For this review, take the finished solid that the model builds, in its own axes (mm). Face numbers are marked on the shaded views. A direction names the side the tool comes from. Give positions to 0.01 mm unless a question says otherwise; leave off trailing zeros. Write each loop counter-clockwise with the first axis right and the second up, starting at its lowest first coordinate (ties: lowest second). Pieces come first, ordered by that corner, then holes. Notation, with made-up numbers: (89.25, 63.5) -> (134.25, 63.5) arc R28 ccw to (134.25, 84.5) -> close; hole circle Ø8 at (72.5, 43). An arc over 180 degrees is marked (long way). Return JSON: item names as keys, results as strings.
from build123d import *

# Parameters (mm, degrees)
SKETCH1_W           = 12
SKETCH1_H           = 16
SKETCH1_R           = 2.1
SKETCH1_W_2         = 2
BOSS_EXTRUDE1_DEPTH = 20
FILLET1_R           = 5
SKETCH2_W           = 9
SKETCH2_H           = 1.9
BOSS_EXTRUDE2_DEPTH = 5


with BuildPart() as part:
    # Sketch1 → Boss-Extrude1 (new body)
    # profile 1 of 2: a face of its own
    with BuildSketch(Plane(origin=(0, 0, 0), x_dir=(1, 0, 0), z_dir=(0, 1, 0))):
        Rectangle(SKETCH1_W, SKETCH1_H)
        with Locations(Location((0, 0, 0), (0, 0, 270))):
            Circle(SKETCH1_R, mode=Mode.SUBTRACT)
    # profile 2 of 2: a face of its own
    with BuildSketch(Plane(origin=(0, 0, 0), x_dir=(1, 0, 0), z_dir=(0, 1, 0))):
        with Locations((7, 0)):
            Rectangle(SKETCH1_W_2, SKETCH1_H)
    extrude(amount=BOSS_EXTRUDE1_DEPTH)

    # Fillet1
    fillet1_edges = [part.edges().sort_by_distance(p)[0] for p in [
        (-6, 10, 8),
        (-6, 10, -8),
    ]]
    fillet(fillet1_edges, radius=FILLET1_R)

    # Sketch2 → Boss-Extrude2 (add)
    with BuildSketch(Plane(origin=(0, 20, 0), x_dir=(1, 0, 0), z_dir=(0, 1, 0))):
        with Locations((3.5, 7.05)):
            Rectangle(SKETCH2_W, SKETCH2_H)
        with Locations((3.5, -7.05)):
            Rectangle(SKETCH2_W, SKETCH2_H)
    extrude(amount=BOSS_EXTRUDE2_DEPTH)


solid = part.part
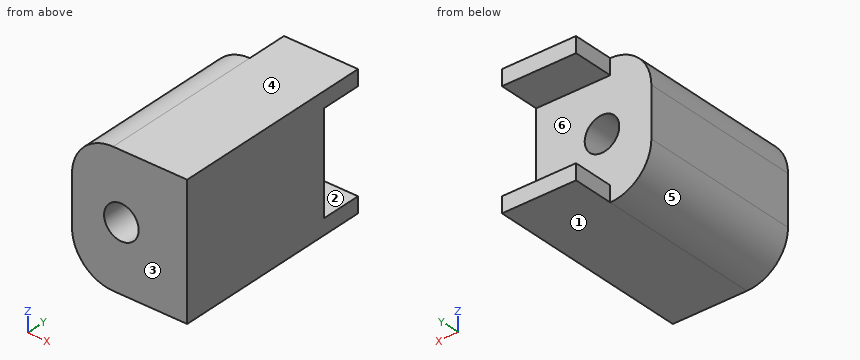
1. For pin 1 (2 mm diameter, centred on y = 22.5, z = 7.5, fed in from -X); pin 2 (2.5 mm diameter, centred on x = 0, z = 0, fed in from -Y), all flat-tipped, find the tip position at first contact; note any pin that passes through.
Results found:
{"pin 1": "stops at x = -1", "pin 2": "passes through"}
2. Add section B-B, the plane y = 6. State the section outline as (x, z) points.
Results found:
{"outline": "(-6, -3) arc R5 ccw to (-1, -8) -> (8, -8) -> (8, 8) -> (-1, 8) arc R5 ccw to (-6, 3) -> close; hole circle Ø4.2 at (0, 0)"}
3. For the marked faces 1 and 2, list the 3-axis set-ups (+Z, -Z, +X, -X, +Y, -Y) from which the entire face can be reached by the end or side of a thin tool; tool diameter is ignored.
Results found:
{"face 1": "-Z, +X, -X, +Y, -Y", "face 2": "+X, -X, +Y"}
4. Add section A-A, the plane z = 0. State the section outline as (x, y) points, plus the area to 3 significant figures.
Results found:
{"outline": "(-6, 0) -> (-2.1, 0) -> (-2.1, 20) -> (-6, 20) -> close; (2.1, 0) -> (8, 0) -> (8, 20) -> (2.1, 20) -> close", "area": "196 mm²"}
5. Add section D-D, the plane y = 21.5. State the section outline as (x, z) points.
Results found:
{"outline": "(-1, -8) -> (8, -8) -> (8, -6.1) -> (-1, -6.1) -> close; (-1, 6.1) -> (8, 6.1) -> (8, 8) -> (-1, 8) -> close"}
6. The part is to be moulded in two halves that separate along Z. For the marked faces 3, 4, 5 and 6, say which applies: +Z half, -Z half, draft (parallel to the pull), parting line (faces both ways), or undercut.
Results found:
{"face 3": "draft", "face 4": "+Z half", "face 5": "-Z half", "face 6": "undercut"}
7. To check wall thickness, follow probe 1 along X at (y, z) = (9.75, 0); probe 2 along Y at (x, z) = (6.5, 4.75); probe 3 along Z at (x, y) = (-1, 13). State the ranges of each line that lie inside material, in increasing order.
Results found:
{"probe 1": "x = -6 to -2.1, 2.1 to 8", "probe 2": "y = 0 to 20", "probe 3": "z = -8 to -1.85, 1.85 to 8"}
8. Add section C-C, the plane x = 0. State the section outline as (y, z) points.
Results found:
{"outline": "(0, -8) -> (25, -8) -> (25, -6.1) -> (20, -6.1) -> (20, -2.1) -> (0, -2.1) -> close; (0, 2.1) -> (20, 2.1) -> (20, 6.1) -> (25, 6.1) -> (25, 8) -> (0, 8) -> close"}
